For this review, use the dimensioned drawing (mm, ordinates from the lowest corner) and the shaded views. A direction names the side the tool comes from. Coordinates: 2 decimals unless noted, no trailing zeros. Order: outer loops, then holes, each group sorted by start corner. A loop starts at its lowest first (then second) coordinate and runs counter-clockwise, first axis right, second up. Notation, with made-up numbers: (-10.5, 35) -> (24.5, 35) arc R35 ccw to (24.5, 69) -> close; hole circle Ø8 at (-15, 24). An arc over 180 degrees is marked (long way). Return JSON: item names as keys, results as strings. Group by question number.
Item 1: Take a section at B-B (x = 4.6). Write out the cut boundary in (y, z), then the cut area to 4 significant figures.
Item 2: Insertion check: pin 1 (2.5 mm diameter, centred on x = 4.6, z = 6.6, fed in from -Y); pin 2 (0.9 mm diameter, centred on x = 27, y = 1, fed in from +Z); pin 3 (1.5 mm diameter, centred on y = 2, z = 27, fed in from -X). Each pin has a flat end and moves straight along its axis. Give the tip position at first contact, or say it passes through.
Item 3: Machinability: for the marked faces 1 and 2, which of the approach directions +Z, -Z, +X, -X, +Y, -Y give a long, thin tool a straight path to every point of the face, cutting with its end or side? Answer none if there is none.
Item 4: Take a section at D-D (z = 24). Write out the cut boundary in (x, y).
Item 5: Take a section at C-C (z = 6.6). Write out the cut boundary in (x, y), then the cut area to 3 significant figures.
Item 6: Draft analysis for pull direction Z (two halves, no side actions). For the marked faces 3, 4 and 5, state which applies: +Z half, -Z half, draft (parallel to the pull), parting line (faces both ways), or undercut.
Item 7: For line 1 along X through (y, z) = (2.1, 6.6); line 2 along Z through (x, y) = (30, 1.55); line 3 along X through (y, z) = (2.8, 9.75), list the stretches that pass through material, from the lowest coordinate up.
Item 8: Take a section at A-A (y = 0.75). Write out the cut boundary in (x, z), then the cut area to 3 significant figures.
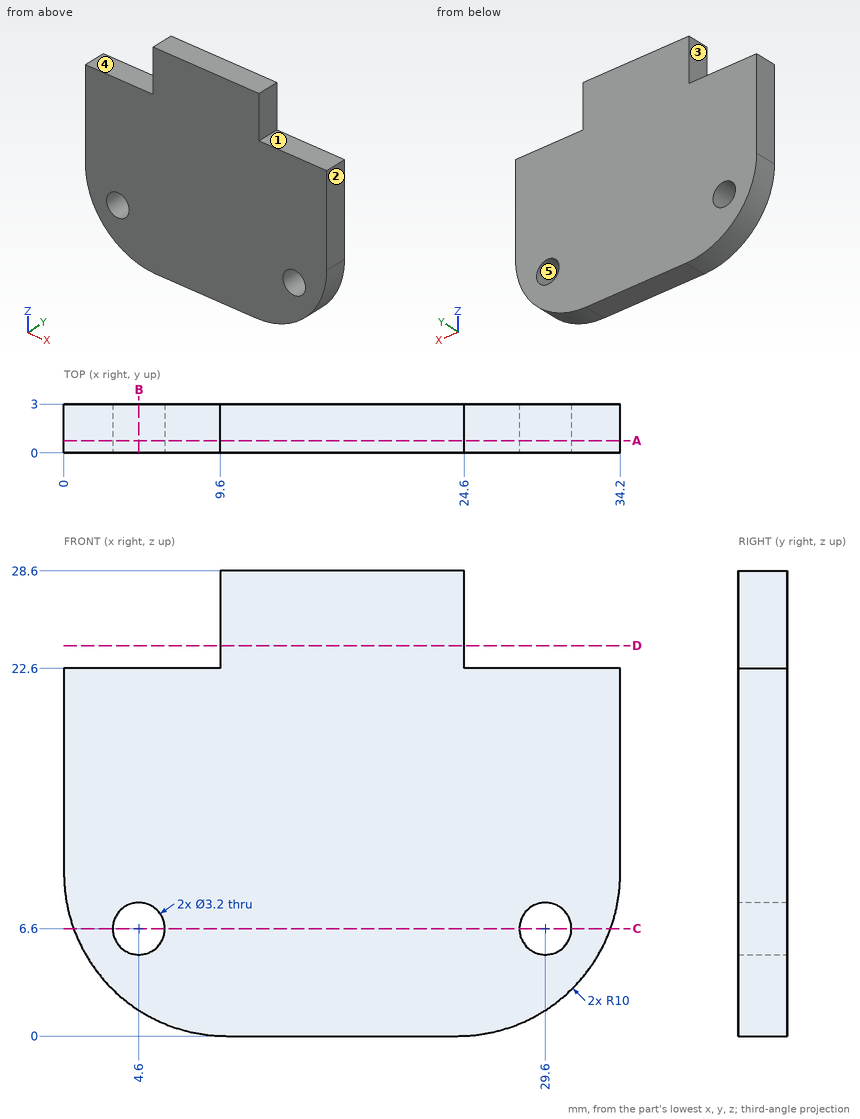
Findings below:
{
 "1": {"outline": "(0, 1.58) -> (3, 1.58) -> (3, 5) -> (0, 5) -> close; (0, 8.2) -> (3, 8.2) -> (3, 22.6) -> (0, 22.6) -> close", "area": "53.45 mm2"},
 "2": {"pin 1": "passes through", "pin 2": "stops at z = 22.6", "pin 3": "stops at x = 9.6"},
 "3": {"face 1": "+Z, +X, +Y, -Y", "face 2": "+Z, -Z, +X, +Y, -Y"},
 "4": {"outline": "(9.6, 0) -> (24.6, 0) -> (24.6, 3) -> (9.6, 3) -> close"},
 "5": {"outline": "(0.6, 0) -> (3, 0) -> (3, 3) -> (0.6, 3) -> close; (6.2, 0) -> (28, 0) -> (28, 3) -> (6.2, 3) -> close; (31.2, 0) -> (33.6, 0) -> (33.6, 3) -> (31.2, 3) -> close", "area": "79.8 mm2"},
 "6": {"face 3": "draft", "face 4": "+Z half", "face 5": "undercut"},
 "7": {"line 1": "x = 0.6 to 3, 6.2 to 28, 31.2 to 33.6", "line 2": "z = 1.85 to 5.05, 8.15 to 22.6", "line 3": "x = 0 to 34.2"},
 "8": {"outline": "(0, 10) arc R10 ccw to (10, 0) -> (24.2, 0) arc R10 ccw to (34.2, 10) -> (34.2, 22.6) -> (24.6, 22.6) -> (24.6, 28.6) -> (9.6, 28.6) -> (9.6, 22.6) -> (0, 22.6) -> close; hole circle Ø3.2 at (4.6, 6.6); hole circle Ø3.2 at (29.6, 6.6)", "area": "804 mm2"}
}
